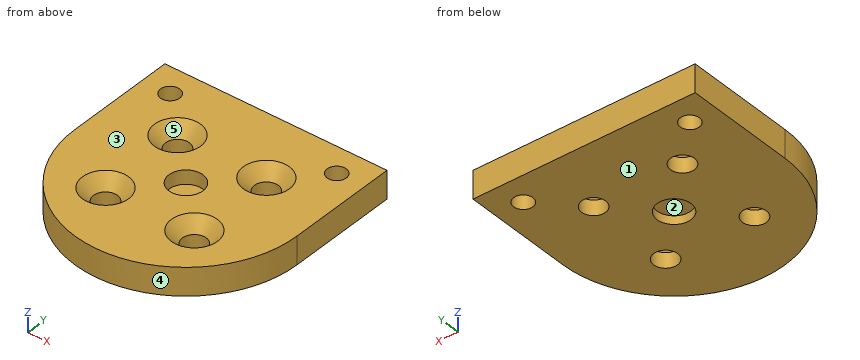
```python
from build123d import *

# Parameters (mm, degrees)
SKETCH104_R         = 3.05
SKETCH104_R_2       = 1.7272
PAD063_DEPTH        = 5
HOLE008_D           = 4.3
HOLE008_CSINK_D     = 8.298
HOLE008_CSINK_ANGLE = 82
SKETCH106_R         = 3.5
PAD064_DEPTH        = 1


with BuildPart() as part:
    # Sketch104 → Pad063 (new body)
    with BuildSketch(Plane.XY):
        with BuildLine():
            ThreePointArc((-20, 0), (0, -20), (20, 0))
            Line((20, 20), (20, 0))
            Line((-20, 20), (20, 20))
            Line((-20, 0), (-20, 20))
        make_face()
        Circle(SKETCH104_R, mode=Mode.SUBTRACT)
        with Locations((-15, 15)):
            Circle(SKETCH104_R_2, mode=Mode.SUBTRACT)
        with Locations((15, 15)):
            Circle(SKETCH104_R_2, mode=Mode.SUBTRACT)
    extrude(amount=PAD063_DEPTH)

    # Hole008 (through all)
    with Locations(Plane.XY.offset(5)):
        with Locations((-8, 8), (8, 8), (8, -8), (-8, -8)):
            CounterSinkHole(HOLE008_D / 2, HOLE008_CSINK_D / 2, counter_sink_angle=HOLE008_CSINK_ANGLE)

    # Sketch106 → Pad064 (join)
    with BuildSketch(Plane.XY.offset(1.5)):
        Circle(SKETCH106_R)
    extrude(amount=PAD064_DEPTH)


solid = part.part
```
Design review of the part built by this model. Coordinates are the model's own, in mm. Face numbers are marked on the shaded views. A direction names the side the tool comes from. Coordinates: 2 decimals unless noted, no trailing zeros. Order: outer loops, then holes, each group sorted by start corner. A loop starts at its lowest first (then second) coordinate and runs counter-clockwise, first axis right, second up. Notation, with made-up numbers: (32.25, -23.75) - (83.25, -23.75) arc R26 cw to (83.25, -8.75) - close; hole circle Ø6 at (-14.75, -39.5). An arc over 180 degrees is marked (long way). Answer in a Markdown table with one row per item.
(1) Wall thickness on line 1 along X through (y, z) = (8, 0.8); line 2 along X through (y, z) = (6.5, 4.7); line 3 along Y through (x, z) = (8, 2.05): over which ranges is each line inside the solid? List them lowest first. Write a range as from..to.
Checked values:
| item | result |
|---|---|
| line 1 | -20..-10.15, -5.85..5.85, 10.15..20 |
| line 2 | -20..-11.59, -4.41..4.41, 11.59..20 |
| line 3 | -18.33..-10.15, -5.85..5.85, 10.15..20 |
(2) Consider section C-C on x = 8. State the section outline as (y, z) points.
Checked values:
| item | result |
|---|---|
| outline | (-18.33, 0) - (-10.15, 0) - (-10.15, 2.7) - (-12.15, 5) - (-18.33, 5) - close; (-5.85, 0) - (5.85, 0) - (5.85, 2.7) - (3.85, 5) - (-3.85, 5) - (-5.85, 2.7) - close; (10.15, 0) - (20, 0) - (20, 5) - (12.15, 5) - (10.15, 2.7) - close |
(3) For the marked faces 1 and 2, list the 3-axis set-ups (+Z, -Z, +X, -X, +Y, -Y) from which the entire face can be reached by the end or side of a thin tool; tool diameter is ignored.
Checked values:
| item | result |
|---|---|
| face 1 | -Z, +X, -X, +Y, -Y |
| face 2 | -Z |
(4) The part is to be moulded in two halves that separate along X. For the marked faces 3, 4 and 5, say which applies: released by +X, released by -X, zero draft, split by the parting line, or undercut.
Checked values:
| item | result |
|---|---|
| face 3 | zero draft |
| face 4 | split by the parting line |
| face 5 | undercut |
(5) Consider section D-D on x = 15. State the section outline as (y, z) points, plus the area to 3 significant figures.
Checked values:
| item | result |
|---|---|
| outline | (-13.23, 0) - (13.27, 0) - (13.27, 5) - (-13.23, 5) - close; (16.73, 0) - (20, 0) - (20, 5) - (16.73, 5) - close |
| area | 149 mm^2 |
(6) Consider section A-A on y = 8. State the section outline as (x, z) points, plus the area to 3 significant figures.
Checked values:
| item | result |
|---|---|
| outline | (-20, 0) - (-10.15, 0) - (-10.15, 2.7) - (-12.15, 5) - (-20, 5) - close; (-5.85, 0) - (5.85, 0) - (5.85, 2.7) - (3.85, 5) - (-3.85, 5) - (-5.85, 2.7) - close; (10.15, 0) - (20, 0) - (20, 5) - (12.15, 5) - (10.15, 2.7) - close |
| area | 148 mm^2 |
(7) Clearance check with flat-ended pins moving along their axes: pin 1 (3 mm diameter, centred on x = 15, y = 15, fed in from -Z); pin 2 (3 mm diameter, centred on x = -1, y = -1, fed in from -Z); pin 3 (3.5 mm diameter, centred on x = 0, y = 0, fed in from +Z). State where each tip first meets the part, or that it passes through.
Checked values:
| item | result |
|---|---|
| pin 1 | through |
| pin 2 | z = 1.5 |
| pin 3 | z = 2.5 |
(8) Consider section B-B on z = 4.35. State the section outline as (x, y) points.
Checked values:
| item | result |
|---|---|
| outline | (-20, 0) arc R20 ccw to (20, 0) - (20, 20) - (-20, 20) - close; hole circle Ø3.45 at (-15, 15); hole circle Ø7.17 at (-8, -8); hole circle Ø7.17 at (-8, 8); hole circle Ø6.1 at (0, 0); hole circle Ø7.17 at (8, -8); hole circle Ø7.17 at (8, 8); hole circle Ø3.45 at (15, 15) |
